```python
from build123d import *

# Parameters (mm, degrees)
BOSS_EXTRU_1_DEPTH      = 6
ESQUISSE2_R             = 4
ESQUISSE2_R_2           = 9
ESQUISSE2_W             = 6
ESQUISSE2_H             = 30
ESQUISSE2_H_2           = 20
ESQUISSE2_W_2           = 12.5
ESQUISSE2_H_3           = 28.5
ENL_V_MAT_EXTRU_1_DEPTH = 6
ESQUISSE3_R             = 1.5
ENL_V_MAT_EXTRU_2_DEPTH = 6
ESQUISSE4_R             = 2.995
ESQUISSE4_R_2           = 3
ENL_V_MAT_EXTRU_3_DEPTH = 3


with BuildPart() as part:
    # Esquisse1 → Boss.-Extru.1 (new body)
    with BuildSketch(Plane.XY):
        Polygon((0, 0), (48, 0), (48, 6), (158, 6), (158, 36), (164, 36), (164, 61), (158, 61), (115, 101.002661161), (-117, 101.002661161), (-160, 61), (-166, 61), (-166, 40), (-110, 40), (-110, 6), (0, 6), align=None)
    extrude(amount=BOSS_EXTRU_1_DEPTH)

    # Esquisse2 → Enlèv. mat.-Extru.1 (cut)
    with BuildSketch(Plane(origin=(0, 0, 0), x_dir=(-1, 0, 0), z_dir=(0, 0, -1))):
        with Locations((-138, 36)):
            Circle(ESQUISSE2_R)
        with Locations((-138, 61)):
            Circle(ESQUISSE2_R_2)
        with Locations((38, 31)):
            Rectangle(ESQUISSE2_W, ESQUISSE2_H)
        with Locations((-36, 31)):
            Rectangle(ESQUISSE2_W, ESQUISSE2_H)
        with Locations((-115, 26)):
            Rectangle(ESQUISSE2_W, ESQUISSE2_H_2)
        with Locations((-111.75, 65.25)):
            Rectangle(ESQUISSE2_W_2, ESQUISSE2_H_3)
    extrude(amount=-ENL_V_MAT_EXTRU_1_DEPTH, mode=Mode.SUBTRACT)

    # Esquisse3 → Enlèv. mat.-Extru.2 (cut)
    with BuildSketch(Plane(origin=(0, 0, 0), x_dir=(-1, 0, 0), z_dir=(0, 0, -1))):
        with Locations((-161, 48.5)):
            Circle(ESQUISSE3_R)
        with Locations((-41, 3)):
            Circle(ESQUISSE3_R)
        with Locations((-7, 3)):
            Circle(ESQUISSE3_R)
        with Locations((-36, 9)):
            Circle(ESQUISSE3_R)
        with Locations((-36, 53)):
            Circle(ESQUISSE3_R)
        with Locations((38, 9)):
            Circle(ESQUISSE3_R)
        with Locations((38, 53)):
            Circle(ESQUISSE3_R)
        with Locations((163, 50.5)):
            Circle(ESQUISSE3_R)
    extrude(amount=-ENL_V_MAT_EXTRU_2_DEPTH, mode=Mode.SUBTRACT)

    # Esquisse4 → Enlèv. mat.-Extru.3 (cut)
    with BuildSketch(Plane(origin=(0, 0, 0), x_dir=(-1, 0, 0), z_dir=(0, 0, -1))):
        with Locations((38, 9)):
            Circle(ESQUISSE4_R)
        with Locations((38, 53)):
            Circle(ESQUISSE4_R_2)
        with Locations((-36, 53)):
            Circle(ESQUISSE4_R_2)
        with Locations((-36, 9)):
            Circle(ESQUISSE4_R_2)
        with Locations((-7, 3)):
            Circle(ESQUISSE4_R)
        with Locations((-41, 3)):
            Circle(ESQUISSE4_R)
        with Locations((-161, 48.5)):
            Circle(ESQUISSE4_R)
        with Locations((163, 50.5)):
            Circle(ESQUISSE4_R)
    extrude(amount=-ENL_V_MAT_EXTRU_3_DEPTH, mode=Mode.SUBTRACT)


solid = part.part
```
Work out the finished part from the listing and answer in its coordinate system (mm). A direction names the side the tool comes from. Coordinates: 2 decimals unless noted, no trailing zeros. Write each loop counter-clockwise with the first axis right and the second up, starting at its lowest first coordinate (ties: lowest second). Pieces come first, ordered by that corner, then holes.
Q1. Each of these flat-tipped pins is pushed along its axis until it touches: pin 1 Ø5.5 at (x, y) = (7, 3) entering from -Z; pin 2 Ø1 at (y, z) = (19, 4.5) entering from +X; pin 3 Ø1.8 at (y, z) = (32.5, 3) entering from -X. Where does it stop, or does it pass through?
Q2. Determine the mould class of faces 1 (the face through (-163, 61, 3)), 2 (the face through (36, 16, 3)), 3 (the face through (24, 0, 3)), 4 (the face through (-3, 51, 0)) for opening direction Y: released by +Y, released by -Y, zero draft, split by the parting line, or undercut.
Q3. A cutting plane is placed at A-A, the plane x = 138. Give the vertices of the cut face in (y, z).
Q4. Find the intervals of material crossed by line 1 (Y direction, x = 36, z = 3.75); line 2 (X direction, y = 36.5, z = 3.85); line 3 (X direction, y = 40.5, z = 1.9), in increasing order.
Q5. A cutting plane is placed at B-B, the plane z = 3.9. State how many separate pieces and enclosed holes the cut face has, then the cut area to 3 significant figures.
Q6. Which of the six approach directions +Z, -Z, +X, -X, +Y, -Y give full straight-line access (tool end or side, diameter ignored) to faces 5 (the face through (115, 36, 3)), 6 (the face through (5.7, 1.7, 3)), 7 (the face through (161, 61, 3)), 8 (the face through (-56, 6, 3))?
Q7. A cutting plane is placed at C-C, the plane x = -63.5. Give the vertices of the cut face in (y, z).
Findings below:
1. pin 1: stops at z = 3
1. pin 2: stops at x = 158
1. pin 3: stops at x = -110
2. face 1: released by +Y
2. face 2: undercut
2. face 3: released by -Y
2. face 4: zero draft
3. outline: (6, 0) - (32, 0) - (32, 6) - (6, 6) - close; (40, 0) - (52, 0) - (52, 6) - (40, 6) - close; (70, 0) - (79.61, 0) - (79.61, 6) - (70, 6) - close
4. line 1: y = 0 to 7.5, 10.5 to 16, 46 to 51.5, 54.5 to 101
4. line 2: x = -110 to -41, -35 to 33, 39 to 134.03, 141.97 to 164
4. line 3: x = -166 to -41, -35 to 33, 39 to 164
5. separate pieces: 1
5. enclosed holes: 14
5. area: 26,200 mm2
6. face 5: +Z, -Z
6. face 6: -Z
6. face 7: +Z, -Z, +X, +Y
6. face 8: +Z, -Z, -X, -Y
7. outline: (6, 0) - (101, 0) - (101, 6) - (6, 6) - close
